from build123d import *

# Parameters (mm, degrees)
F0_W      = 40
F0_H      = 131.9999998143
F1_DEPTH  = 5
F2_W      = 40
F2_H      = 2
F3_DEPTH  = 15
F4_D      = 5.5
F4_DEPTH  = 8
F4_TIP    = 1.6523667023
F5_SIZE   = 1
F6_W      = 40
F6_H      = 25
F7_DEPTH  = 6
F8_R      = 2
F9_DEPTH  = 5
F10_SIZE  = 5.99999
F11_R     = 4
F12_D     = 2.8
F12_DEPTH = 8
F12_TIP   = 0.8412048666
F13_W     = 1.5
F13_H     = 18
F14_DEPTH = 1
F15_SIZE  = 0.99999


# Not quite as in the source:
# - a fillet or chamfer is up to 0.001 mm smaller than in the source, because OpenCascade refuses the exact size


with BuildPart() as f1:
    # F0 (on Top) → F1 (new body)
    with BuildSketch(Plane.XY):
        with Locations((0, 9.28e-08)):
            Rectangle(F0_W, F0_H)
    extrude(amount=F1_DEPTH)

    # F2 (on face) → F3 (join)
    with BuildSketch(Plane.XY.offset(5)):
        with Locations((0, -64.9999998143)):
            Rectangle(F2_W, F2_H)
    extrude(amount=F3_DEPTH)

    # F4
    with Locations(Plane.XY.offset(5)):
        with Locations((-15, -21.9999998143), (15, -21.9999998143)):
            Hole(F4_D / 2, depth=F4_DEPTH)
            with Locations((0, 0, -(F4_DEPTH + F4_TIP / 2))):  # 118° drill point
                Cone(0, F4_D / 2, F4_TIP, mode=Mode.SUBTRACT)

    # F5
    f5_edges = [f1.edges().sort_by_distance(p)[0] for p in [
        (0, -66, 20),
        (0, -66, 0),
        (-17.75, -22, 0),
        (12.25, -22, 0),
    ]]
    chamfer(f5_edges, length=F5_SIZE)

    # F6 (on face) → F7 (join)
    with BuildSketch(Plane.XY.offset(5)):
        with Locations((0, 41.5)):
            Rectangle(F6_W, F6_H)
    extrude(amount=F7_DEPTH)

    # F8 (on face) → F9 (cut)
    with BuildSketch(Plane(origin=(0, 54, 0), x_dir=(-1, 0, 0), z_dir=(0, 1, 0))):
        with Locations((-15, 7.5)):
            Circle(F8_R)
        with Locations((15, 7.5)):
            Circle(F8_R)
    extrude(amount=-F9_DEPTH, mode=Mode.SUBTRACT)

    # F10 (size 6 in the source; OpenCascade refuses exactly that, so slightly less here)
    f10_edges = [f1.edges().sort_by_distance(p)[0] for p in [
        (0, 29, 11),
    ]]
    chamfer(f10_edges, length=F10_SIZE)

    # F11
    f11_edges = [f1.edges().sort_by_distance(p)[0] for p in [
        (-20, 44.499995, 11),
        (20, 44.499995, 11),
    ]]
    fillet(f11_edges, radius=F11_R)

    # F12
    with Locations(Plane.XY.offset(5)):
        with Locations((10, 61), (-10, 61)):
            Hole(F12_D / 2, depth=F12_DEPTH)
            with Locations((0, 0, -(F12_DEPTH + F12_TIP / 2))):  # 118° drill point
                Cone(0, F12_D / 2, F12_TIP, mode=Mode.SUBTRACT)

    # F13 (on face) → F14 (join)
    with BuildSketch(Plane.XZ.offset(65.9999998143)):
        with Locations((-19.25, 10)):
            Rectangle(F13_W, F13_H)
        with Locations((19.25, 10)):
            Rectangle(F13_W, F13_H)
    extrude(amount=F14_DEPTH)

    # F15 (size 1 in the source; OpenCascade refuses exactly that, so slightly less here)
    f15_edges = [f1.edges().sort_by_distance(p)[0] for p in [
        (-19.25, -67, 19),
        (-19.25, -67, 1),
        (19.25, -67, 19),
        (19.25, -67, 1),
    ]]
    chamfer(f15_edges, length=F15_SIZE)


solid = f1.part
The listing builds one solid part. Answer for the finished solid, in the listing's coordinates (mm). A direction names the side the tool comes from. Round coordinates to 2 decimals unless told otherwise and drop trailing zeros. Write each loop counter-clockwise with the first axis right and the second up, starting at its lowest first coordinate (ties: lowest second). Pieces come first, ordered by that corner, then holes. Notation, with made-up numbers: M -28,55 L -16,55 A19 ccw -16,82 Z; hole C -34,38.25 d5. An arc over 180 degrees is marked long. Write each question's results on one line, items separated by ' | '. Start each with the question number.
(1) Each of these flat-tipped pins is pushed along its axis until it touches: P1, Ø8, axis at x = -10, y = 36.5, coming from the +Z side; P2, Ø6, axis at x = -5, y = 27.5, coming from the +Z side; P3, Ø3, axis at x = -3.5, z = 4.5, coming from the -Y side. Where does it stop, or does it pass through?
(2) The part is cut by section C-C, the plane z = 14.5. Write down the section's boundary in (x, y), and give its area (3 significant figures).
(3) The part is cut by section A-A, the plane y = -22. Write down the section's boundary in (x, z), and give its area (3 significant figures).
(4) For faces 4 (the flat face through (0, 45, 11)), 5 (the flat face through (0, -64, 12)), 6 (the flat face through (-15, 49, 8)), 7 (the cylindrical face through (-8.6, 61.06, 2.46)), 8 (the flat face through (20, -6, 4)), determine the directions among +Z, -Z, +X, -X, +Y, -Y from which every point of the face is accessible in a straight line to the end or side of a thin tool.
(5) Find the intervals of material crossed by line 1 (Y direction, x = -15, z = 2.65); line 2 (Y direction, x = 10, z = 3.95); line 3 (X direction, y = 51.5, z = 6.75), in increasing order.
(6) Determine the mould class of faces 1 (the flat face through (-20, -5, 4)), 2 (the cylindrical face through (18.797, 42.661, 9.859)), 3 (the cylindrical face through (15.26, 51.535, 9.483)) for opening direction Z: +Z half, -Z half, draft (parallel to the pull), parting line (faces both ways), or undercut.
Worked answers:
1) P1: stops at z = 11 | P2: stops at z = 6.5 | P3: stops at y = -66
2) outline: M -20,-67 L -18.5,-67 L -18.5,-66 L 18.5,-66 L 18.5,-67 L 20,-67 L 20,-64 L -20,-64 Z | area: 83.0 mm²
3) outline: M -20,0 L -18.75,0 L -17.75,1 L -17.75,5 L -20,5 Z; M -12.25,1 L -11.25,0 L 11.25,0 L 12.25,1 L 12.25,5 L -12.25,5 Z; M 17.75,1 L 18.75,0 L 20,0 L 20,5 L 17.75,5 Z | area: 143 mm²
4) face 4: +Z, +X, -X, +Y | face 5: +Z, +X, -X | face 6: +Y | face 7: +Z, -Z | face 8: +Z, -Z, +X, +Y, -Y
5) line 1: y = -66 to -24.75, -19.25 to 66 | line 2: y = -66 to 59.6, 62.4 to 66 | line 3: x = -20 to -16.85, -13.15 to 13.15, 16.85 to 20
6) face 1: draft | face 2: +Z half | face 3: undercut
